from build123d import *

# Parameters (mm, degrees)
F0_W     = 117.5417516827
F0_H     = 12.7
F0_H_2   = 12.9770076108
F1_DEPTH = 254


with BuildPart() as f1:
    # F0 (on Top) → F1 (new body)
    with BuildSketch(Plane.XY):
        Polygon((-71.8018082797, 70.6772367408), (-71.8018082797, -71.4734956291), (-59.1018082797, -71.4734956291), (-59.1018082797, -58.7734956291), (-59.1018082797, 57.70022913), (-59.1018082797, 70.6772367408), align=None)
        with Locations((-0.3309324384, -65.1234956291)):
            Rectangle(F0_W, F0_H)
        Polygon((58.439943403, -58.7734956291), (58.439943403, -71.4734956291), (58.439943403, -71.8612532069), (71.139943403, -71.8612532069), (71.139943403, 70.6772367408), (58.439943403, 70.6772367408), (58.439943403, 57.70022913), align=None)
        with Locations((-0.3309324384, 64.1887329354)):
            Rectangle(F0_W, F0_H_2)
    extrude(amount=F1_DEPTH)


solid = f1.part
Work out the finished part from the listing and answer in its coordinate system (mm). A direction names the side the tool comes from. Coordinates: 2 decimals unless noted, no trailing zeros. Write each loop counter-clockwise with the first axis right and the second up, starting at its lowest first coordinate (ties: lowest second). Pieces come first, ordered by that corner, then holes. Notation, with made-up numbers: M 71.25,41.5 L 87.25,41.5 A8 ccw 87.25,54.5 Z; hole C 55.5,-16 d8. An arc over 180 degrees is marked long. Use one line per item in the form item = value. Start each with the question number.
1. The part is cut by section A-A (x = 38). Give the vertices of the cut face in (y, z), plus the area to 3 significant figures.
2. Straight lines are drawn through the part: probe 1 along Y at (x, z) = (-11, 188); probe 2 along X at (y, z) = (13.5, 150); probe 3 along Y at (x, z) = (-59.5, 42). For each, find the intervals that lie inside material, in ascending order. Write a range as from..to.
3. A tool of negligible diameter and unlimited length cuts with its end or side. For faces 1 (the face through (65, -71.861, 125)), 2 (the face through (-1, 57.7, 125)), from which of +Z, -Z, +X, -X, +Y, -Y can it reach the whole face along a straight path? Write none if from no direction.
4. The part is cut by section C-C (z = 118.5). Give the vertices of the cut face in (x, y).
5. This flat-tipped pin is pushed along its axis until it touches: P1, Ø5, axis at x = 34.5, z = 177, coming from the -Y side. Where does it stop, or does it pass through?
6. The mould has two halves that part along Y. Classify faces 3 (the face through (-71.802, 1, 125)), 4 (the face through (58.44, 0, 125)), 5 (the face through (-8, -71.473, 125)): released by +Y, released by -Y, zero draft, split by the parting line, or undercut.
7. The part is cut by section B-B (y = -7). Give the vertices of the cut face in (x, z), plus the area to 3 significant figures.
Evaluation:
q1.outline = M -71.47,0 L -58.77,0 L -58.77,254 L -71.47,254 Z; M 57.7,0 L 70.68,0 L 70.68,254 L 57.7,254 Z
q1.area = 6,520 mm^2
q2.probe_1 = -71.47..-58.77, 57.7..70.68
q2.probe_2 = -71.8..-59.1, 58.44..71.14
q2.probe_3 = -71.47..70.68
q3.face_1 = +Z, -Z, +X, -X, -Y
q3.face_2 = +Z, -Z
q4.outline = M -71.8,-71.47 L 58.44,-71.47 L 58.44,-71.86 L 71.14,-71.86 L 71.14,70.68 L -71.8,70.68 Z; hole M -59.1,-58.77 L 58.44,-58.77 L 58.44,57.7 L -59.1,57.7 Z
q5.P1 = -71.47
q6.face_3 = zero draft
q6.face_4 = undercut
q6.face_5 = released by -Y
q7.outline = M -71.8,0 L -59.1,0 L -59.1,254 L -71.8,254 Z; M 58.44,0 L 71.14,0 L 71.14,254 L 58.44,254 Z
q7.area = 6,450 mm^2
